Could you check a few things on this model? Use its own coordinates, in mm. A direction names the side the tool comes from. Give positions to 0.01 mm unless a question says otherwise; leave off trailing zeros. Loops run counter-clockwise (first coordinate to the right, second up) from the corner with the lowest first, then second, coordinate; pieces in that order, holes last. Notation, with made-up numbers: (-22.75, 44.25) -> (26.25, 44.25) arc R20 cw to (26.25, 57.25) -> close; hole circle Ø7 at (66, 4). An arc over 180 degrees is marked (long way). Put each result on its own line as item: value.
```python
from build123d import *

# Parameters (mm, degrees)
BOSS_EXTRUDE1_DEPTH      = 12
BOSS_EXTRUDE1_DEPTH_BACK = 12
FILLET1_R                = 2
SKETCH4_R                = 2.75
CUT_EXTRUDE1_DEPTH       = 66.1459899
CHAMFER1_SIZE            = 1


with BuildPart() as part:
    # Sketch3 → Boss-Extrude1 (new, two sides: drawn at the far end of the back side and taken through both)
    with BuildSketch(Plane(origin=(0, 0, 0), x_dir=(0, 0, -1), z_dir=(1, 0, 0)).offset(-BOSS_EXTRUDE1_DEPTH_BACK)):
        Polygon((0, 62), (-8, 62), (-8, 0), (0, 0), (16, 16), (16, 62), align=None)
    extrude(amount=BOSS_EXTRUDE1_DEPTH + BOSS_EXTRUDE1_DEPTH_BACK)

    # Fillet1
    fillet1_edges = [part.edges().sort_by_distance(p)[0] for p in [
        (-12, 31, 8),
        (12, 31, 8),
    ]]
    fillet(fillet1_edges, radius=FILLET1_R)

    # Sketch4 → Cut-Extrude1 (cut, through all)
    with BuildSketch(Plane(origin=(0, 62, 0), x_dir=(1, 0, 0), z_dir=(0, 1, 0))):
        with Locations((0, 4)):
            Circle(SKETCH4_R)
        with BuildLine():
            ThreePointArc((1.944543648, 2.055456352), (0, 1.25), (-1.944543648, 2.055456352))
            Line((-1.944543648, 2.055456352), (0, 0.110912703))
            Line((0, 0.110912703), (1.944543648, 2.055456352))
        make_face()
    extrude(amount=-CUT_EXTRUDE1_DEPTH, mode=Mode.SUBTRACT)

    # Chamfer1
    chamfer1_edges = [part.edges().sort_by_distance(p)[0] for p in [
        (0, 62, -6.75),
        (-0.972271824, 62, -1.083184528),
        (0.972271824, 62, -1.083184528),
    ]]
    chamfer(chamfer1_edges, length=CHAMFER1_SIZE)


solid = part.part
```
1. If we section it at C-C (x = 7.25): List the corners of the cut face in (y, z) for me, then the cut area to 3 significant figures.
Recorded:
outline: (0, 0) -> (16, -16) -> (62, -16) -> (62, 8) -> (0, 8) -> close
area: 1,360 mm^2
2. For faces 1 (the face through (-1.3, 61.5, -0.7)), 2 (the face through (-0.99, 30.98, -1.1)), 3 (the face through (0, 8, -8)), which set-ups out of +Z, -Z, +X, -X, +Y, -Y let a thin tool reach every point of the face, with its end or its side?
Recorded:
face 1: +Y
face 2: +Y, -Y
face 3: -Z, +X, -X, -Y
3. If we section it at D-D (z = -11.25): List the corners of the cut face in (x, y) for me.
Recorded:
outline: (-12, 11.25) -> (12, 11.25) -> (12, 62) -> (-12, 62) -> close
4. Thinking about a two-plate mould opening in X: for faces 4 (the face through (0, 31, 8)), 5 (the face through (0.09, 31.94, -6.75)), 6 (the face through (-11.4, 30.57, 7.43)), which applies, pulls with the +X half, pulls with the -X half, needs draft (parallel to the pull), parting line crosses it, or undercut?
Recorded:
face 4: needs draft
face 5: undercut
face 6: pulls with the -X half
5. If we section it at B-B (z = -4): List the corners of the cut face in (x, y) for me, then the cut area to 3 significant figures.
Recorded:
outline: (-12, 4) -> (-2.75, 4) -> (-2.75, 61) -> (-3.75, 62) -> (-12, 62) -> close; (2.75, 4) -> (12, 4) -> (12, 62) -> (3.75, 62) -> (2.75, 61) -> close
area: 1,070 mm^2
6. I'm going to push flat-ended pins straight in: pin 1 (6.5 mm diameter, centred on x = 0, z = -4, fed in from -Y); pin 2 (3 mm diameter, centred on x = 4, y = 10.5, fed in from -Z); pin 3 (2 mm diameter, centred on x = -1.5, z = -5.5, fed in from +Y). Where does each tip first touch, or does it pass through?
Recorded:
pin 1: stops at y = 0.83
pin 2: stops at z = -12
pin 3: stops at y = 61.37
7. I need wall thicknesses on line 1 (X direction, y = 44, z = -4); line 2 (Y direction, x = 0.25, z = -8); line 3 (X direction, y = 11, z = -6). Which ranges of each line are inside material? Lowest first, please.
Recorded:
line 1: x = -12 to -2.75, 2.75 to 12
line 2: y = 8 to 62
line 3: x = -12 to -1.89, 1.89 to 12
8. If we section it at A-A (y = 28): List the corners of the cut face in (x, z) for me, then the cut area to 3 significant figures.
Recorded:
outline: (-12, -16) -> (12, -16) -> (12, 6) arc R2 ccw to (10, 8) -> (-10, 8) arc R2 ccw to (-12, 6) -> close; hole (-1.94, -2.06) arc R2.75 ccw (long way) to (1.94, -2.06) -> (0, -0.11) -> close
area: 549 mm^2
